Could you check a few things on this model? Use its own coordinates, in mm. A direction names the side the tool comes from. Round coordinates to 2 decimals unless told otherwise and drop trailing zeros. Write each loop counter-clockwise with the first axis right and the second up, starting at its lowest first coordinate (ties: lowest second). Pieces come first, ordered by that corner, then holes. Notation, with made-up numbers: (-18, 48) - (36, 48) arc R37 cw to (36, 84) - close; hole circle Ø6 at (40.25, -8). An arc over 180 degrees is marked (long way). Write each question's results on one line, items separated by ' | '. Start each with the question number.
(1) Imagine slicing it at C-C on z = -1.5. Write out the boundary of the cut face in (x, y), then the cut area to 3 significant figures.
(2) Thinking about a two-plate mould opening in Y: for faces 3 (the cylindrical face through (-0.9, 6.84, 0.09)), 4 (the cylindrical face through (14.21, 4.48, 6.5)), 5 (the flat face through (6, -6, -7.25)), which applies, +Y half, -Y half, draft (parallel to the pull), parting line (faces both ways), or undercut?
(3) On a 3-axis mill with a long thin cutter (end or side, diameter ignored), from which of +Z, -Z, +X, -X, +Y, -Y can I reach the whole of each face in a straight line? I mean faces 1 (the conical face through (11.53, 3.63, -4.28)), 2 (the flat face through (6, -6, 7.25)). Say none if no direction works.
(4) For P1, Ø2, axis at x = 0, z = 2, coming from the +Y side; P2, Ø1.5, axis at y = -3, z = -4.5, coming from the -X side; P3, Ø4, axis at x = 11.5, z = -4.5, coming from the -Y side, each with a flat end and sliding along its axis, tell me the tip position at first contact or that it passes through.
(5) Imagine slicing it at A-A on y = 0. Write out the boundary of the cut face in (x, z).
(6) Please list where these lines run through material, in increasing order: line 1 (Y direction, x = 0, z = -2.25); line 2 (Y direction, x = 3.5, z = 6.5); line 3 (Z direction, x = -10.25, y = -8.75). Write a range as [from, to].
```python
from build123d import *

# Parameters (mm, degrees)
SKETCH1_R           = 11.9
SKETCH1_R_2         = 6.9
BOSS_EXTRUDE1_DEPTH = 6.25
SKETCH2_R           = 14.9
SKETCH2_R_2         = 6.9
BOSS_EXTRUDE2_DEPTH = 1
CHAMFER1_SIZE       = 2.100622615
CHAMFER1_SIZE_2     = 3
CHAMFER2_SIZE       = 0.5
CHAMFER3_SIZE       = 1


with BuildPart() as part:
    # Sketch1 → Boss-Extrude1 (new, symmetric)
    with BuildSketch(Plane.XY):
        Circle(SKETCH1_R)
        Circle(SKETCH1_R_2, mode=Mode.SUBTRACT)
    extrude(amount=BOSS_EXTRUDE1_DEPTH, both=True)

    # Sketch2 → Boss-Extrude2 (add)
    with BuildSketch(Plane.XY.offset(6.25)):
        Circle(SKETCH2_R)
        Circle(SKETCH2_R_2, mode=Mode.SUBTRACT)
    boss_extrude2 = extrude(amount=BOSS_EXTRUDE2_DEPTH)

    # Mirror1: Boss-Extrude2 across plane
    add(boss_extrude2.mirror(Plane.XY))

    # Chamfer1
    # the kernel refuses this chamfer: 3, 2.100622615 mm, written as the material it adds along each edge
    with BuildSketch(Plane(origin=(0, 0, -6.25), x_dir=(1, 0, 0), z_dir=(0, -1, 0))) as chamfer1_piece_1_section:
        Polygon((11.9, CHAMFER1_SIZE), (11.9 + CHAMFER1_SIZE_2, 0), (11.9, 0), align=None)
    chamfer1_piece_1 = revolve(axis=Axis((0, 0, -6.25), (0, 0, 1)), mode=Mode.PRIVATE)
    chamfer1_piece_1 = chamfer1_piece_1 & Plane(origin=(0, 0, -5.219213632), x_dir=(1, 0, 0), z_dir=(0, 0, 1)) * Cylinder(14.9, 60, mode=Mode.PRIVATE)
    add(chamfer1_piece_1)
    with BuildSketch(Plane(origin=(0, 0, 6.25), x_dir=(1, 0, 0), z_dir=(0, -1, 0))) as chamfer1_piece_2_section:
        Polygon((11.9, -CHAMFER1_SIZE), (11.9 + CHAMFER1_SIZE_2, 0), (11.9, 0), align=None)
    chamfer1_piece_2 = revolve(axis=Axis((0, 0, 6.25), (0, 0, 1)), mode=Mode.PRIVATE)
    chamfer1_piece_2 = chamfer1_piece_2 & Plane(origin=(0, 0, 5.219213632), x_dir=(1, 0, 0), z_dir=(0, 0, -1)) * Cylinder(14.9, 60, mode=Mode.PRIVATE)
    add(chamfer1_piece_2)

    # Chamfer2
    chamfer2_edges = [part.edges().sort_by_distance(p)[0] for p in [
        (-14.9, 0, 7.25),
        (-14.9, 0, -7.25),
    ]]
    chamfer(chamfer2_edges, length=CHAMFER2_SIZE)

    # Chamfer3
    chamfer3_edges = [part.edges().sort_by_distance(p)[0] for p in [
        (-6.9, 0, 7.25),
        (-6.9, 0, -7.25),
    ]]
    chamfer(chamfer3_edges, length=CHAMFER3_SIZE)


solid = part.part
```
Response:
1) outline: circle Ø23.8 at (0, 0); hole circle Ø13.8 at (0, 0) | area: 295 mm²
2) face 3: undercut | face 4: parting line | face 5: draft
3) face 1: none | face 2: +Z, +X, -X, +Y, -Y
4) P1: y = 11.9 | P2: x = -13.15 | P3: y = -10.54
5) outline: (-14.9, -6.75) - (-14.4, -7.25) - (-7.9, -7.25) - (-6.9, -6.25) - (-6.9, 6.25) - (-7.9, 7.25) - (-14.4, 7.25) - (-14.9, 6.75) - (-14.9, 6.25) - (-11.9, 4.15) - (-11.9, -4.15) - (-14.9, -6.25) - close; (6.9, -6.25) - (7.9, -7.25) - (14.4, -7.25) - (14.9, -6.75) - (14.9, -6.25) - (11.9, -4.15) - (11.9, 4.15) - (14.9, 6.25) - (14.9, 6.75) - (14.4, 7.25) - (7.9, 7.25) - (6.9, 6.25) - close
6) line 1: [-11.9, -6.9], [6.9, 11.9] | line 2: [-14.48, -6.23], [6.23, 14.48] | line 3: [-7.25, -5.25], [5.25, 7.25]
